Autodesk Inventor part; units mm, degrees
ref_plane "YZ Plane" through (0, 0, 0) normal (1, 0, 0) x (0, 1, 0)
ref_plane "XZ Plane" through (0, 0, 0) normal (0, 1, 0) x (-1, 0, 0)
ref_plane "XY Plane" through (0, 0, 0) normal (0, 0, 1) x (1, 0, 0)
sketch "Base" plane through (0, 0, 0) normal (0, 0, 1) x (1, 0, 0)
  circle A0 centre (0, 0) radius 7.75
  line L0 (0, 0) -> (-34, 0) construction
  circle A1 centre (-34, 0) radius 7.75
  circle A2 centre (0, 0) radius 3
  circle A3 centre (-34, 0) radius 3
  line L1 (-34, 7.75) -> (0, 7.75)
  line L2 (-34, -7.75) -> (0, -7.75)
  dimension "d0" = 15.5
  dimension "d1" = 34
  dimension "d3" = 6
extrude "BaseFeature" add sketch "Base" along normal blind 3
properties part number "BackSideConnector"
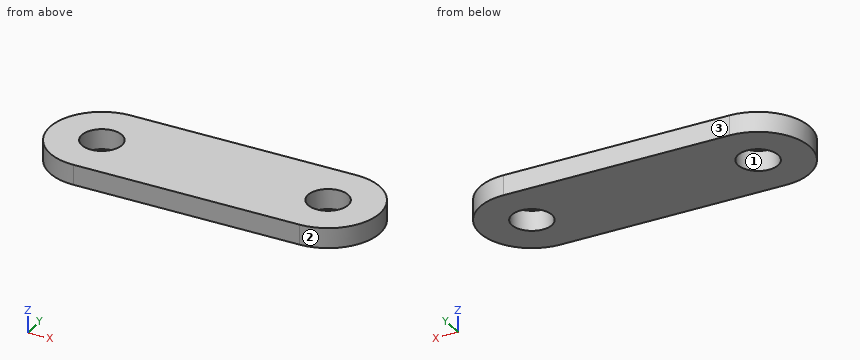
Build history of the part. All positions in model axes, mm. Face numbers are marked on the shaded views. Coordinates: 2 decimals unless noted, no trailing zeros. Order: outer loops, then holes, each group sorted by start corner. A loop starts at its lowest first (then second) coordinate and runs counter-clockwise, first axis right, second up. Notation, with made-up numbers: (-18, -28) -> (7, -28) arc R29 cw to (7, 4) -> close; hole circle Ø6 at (36, 47). An arc over 180 degrees is marked (long way). Answer in a Markdown table with one row per item. Add a question column.
Q1. Band-saw the part on A-A, the plane y = 0. List the corners of the cut face in (x, z), then the cut area to 4 significant figures.
Q2. Band-saw the part on D-D, the plane y = 2.25. List the corners of the cut face in (x, z).
Q3. Wall check: line 1 along Y through (x, z) = (-34, 1.6); line 2 along X through (y, z) = (1.25, 2.5); line 3 along X through (y, z) = (-2.5, 0.95). Give the ranges that are in metal, low to high. Write a range as [from, to].
Q4. Band-saw the part on B-B, the plane z = 1.65. List the corners of the cut face in (x, y).
Q5. Mould opens along X. For the marked faces 1, 2 and 3 say: +X half, -X half, draft (parallel to the pull), parting line (faces both ways), or undercut.
Q6. Band-saw the part on C-C, the plane x = 0.5. List the corners of the cut face in (y, z), then the cut area to 3 significant figures.
Answers follow:
| question | item | result |
|---|---|---|
| 1 | outline | (-41.75, 0) -> (-37, 0) -> (-37, 3) -> (-41.75, 3) -> close; (-31, 0) -> (-3, 0) -> (-3, 3) -> (-31, 3) -> close; (3, 0) -> (7.75, 0) -> (7.75, 3) -> (3, 3) -> close |
| 1 | area | 112.5 mm^2 |
| 2 | outline | (-41.42, 0) -> (-35.98, 0) -> (-35.98, 3) -> (-41.42, 3) -> close; (-32.02, 0) -> (-1.98, 0) -> (-1.98, 3) -> (-32.02, 3) -> close; (1.98, 0) -> (7.42, 0) -> (7.42, 3) -> (1.98, 3) -> close |
| 3 | line 1 | [-7.75, -3], [3, 7.75] |
| 3 | line 2 | [-41.65, -36.73], [-31.27, -2.73], [2.73, 7.65] |
| 3 | line 3 | [-41.34, -35.66], [-32.34, -1.66], [1.66, 7.34] |
| 4 | outline | (-34, -7.75) -> (0, -7.75) arc R7.75 ccw to (0, 7.75) -> (-34, 7.75) arc R7.75 ccw to start; hole circle Ø6 at (-34, 0); hole circle Ø6 at (0, 0) |
| 5 | face 1 | undercut |
| 5 | face 2 | +X half |
| 5 | face 3 | draft |
| 6 | outline | (-7.73, 0) -> (-2.96, 0) -> (-2.96, 3) -> (-7.73, 3) -> close; (2.96, 0) -> (7.73, 0) -> (7.73, 3) -> (2.96, 3) -> close |
| 6 | area | 28.7 mm^2 |
